from build123d import *

# Parameters (mm, degrees)
F1_DEPTH = 41.275
F2_W     = 82.55
F2_H     = 5.08
F3_DEPTH = 5.08
F4_W     = 92.71
F4_H     = 8.89
F5_DEPTH = 5.08
F6_W     = 5.0743944012
F6_H     = 7.62
F7_DEPTH = 6.35
F8_SIZE  = 1.27
F9_SIZE  = 3.048


with BuildPart() as f1:
    # F0 (on Front) → F1 (new body, symmetric)
    with BuildSketch(Plane.XZ):
        Polygon((-41.275, -3.81), (-41.275, 0), (-41.275, 5.08), (-46.355, 5.08), (-46.355, -3.81), align=None)
        Polygon((41.275, 0), (0, 0), (-41.275, 0), (-41.275, -3.81), (41.275, -3.81), align=None)
        Polygon((41.275, 5.08), (41.275, 0), (41.275, -3.81), (46.355, -3.81), (46.355, 5.08), align=None)
    extrude(amount=F1_DEPTH, both=True)

    # F2 (on face) → F3 (join)
    with BuildSketch(Plane.XZ.offset(41.275)):
        Polygon((-46.355, 5.08), (-46.355, -3.81), (46.355, -3.81), (46.355, 5.08), (41.275, 5.08), (41.275, 0), (-41.275, 0), (-41.275, 5.08), align=None)
        with Locations((0, 2.54)):
            Rectangle(F2_W, F2_H)
    extrude(amount=F3_DEPTH)

    # F4 (on face) → F5 (join)
    with BuildSketch(Plane(origin=(0, 41.275, 0), x_dir=(-1, 0, 0), z_dir=(0, 1, 0))):
        with Locations((0, 0.635)):
            Rectangle(F4_W, F4_H)
    extrude(amount=F5_DEPTH)

    # F6 (on face) → F7 (join)
    with BuildSketch(Plane.XZ.offset(46.355)):
        Rectangle(F6_W, F6_H)
    extrude(amount=F7_DEPTH)

    # F8
    f8_edges = [f1.edges().sort_by_distance(p)[0] for p in [
        (-2.537197, -49.53, 3.81),
        (2.537197, -49.53, 3.81),
        (0, -52.705, 3.81),
        (2.537197, -52.705, 0),
        (-2.537197, -52.705, 0),
    ]]
    chamfer(f8_edges, length=F8_SIZE)

    # F9
    f9_edges = [f1.edges().sort_by_distance(p)[0] for p in [
        (-41.275, 0, 5.08),
        (0, 41.275, 5.08),
        (0, -41.275, 5.08),
        (41.275, 0, 5.08),
    ]]
    chamfer(f9_edges, length=F9_SIZE)


solid = f1.part
Work out the finished part from the listing and answer in its coordinate system (mm). A direction names the side the tool comes from. Coordinates: 2 decimals unless noted, no trailing zeros. Write each loop counter-clockwise with the first axis right and the second up, starting at its lowest first coordinate (ties: lowest second). Pieces come first, ordered by that corner, then holes. Notation, with made-up numbers: M -5.75,9 L 26.25,9 A28 ccw 26.25,40 Z; hole C 18,58.25 d1. An arc over 180 degrees is marked long. Use one line per item in the form item = value. Start each with the question number.
1. Straight lines are drawn through the part: probe 1 along X at (y, z) = (15.5, 2) (3 decimals); probe 2 along Z at (x, y) = (-38, -16.5). For each, find the intervals that lie inside material, in ascending order. Write a range as from..to.
2. A tool of negligible diameter and unlimited length cuts with its end or side. For faces 1 (the face through (1, -1, 0)), 2 (the face through (-46.355, -1, 1)), 3 (the face through (2.537, -49, -1)), from which of +Z, -Z, +X, -X, +Y, -Y can it reach the whole face along a straight path? Write none if from no direction.
3. Each of these flat-tipped pins is pushed along its axis until it touches: P1, Ø2.5, axis at y = -49.5, z = -1.5, coming from the -X side; P2, Ø1.3, axis at x = 0.5, y = -50, coming from the +Z side; P3, Ø4, axis at y = -48.5, z = -1, coming from the +X side. Where does it stop, or does it pass through?
4. The part is cut by section A-A (y = -4). Give the vertices of the cut face in (x, z) (3 decimals), plus the area to 3 significant figures.
5. The mould has two halves that part along X. Classify faces 4 (the face through (0, -49, 3.81)), 5 (the face through (-2.537, -49, -1)), 6 (the face through (0.621, 42.778, 3.535)), 7 (the face through (-42.778, 0.621, 3.535)): released by +X, released by -X, zero draft, split by the parting line, or undercut.
Evaluation:
q1.probe_1 = -46.355..-41.275, 41.275..46.355
q1.probe_2 = -3.81..0
q2.face_1 = +Z
q2.face_2 = +Z, -Z, -X, +Y, -Y
q2.face_3 = +Z, -Z, +X, -Y
q3.P1 = -2.54
q3.P2 = 3.81
q3.P3 = 2.54
q4.outline = M -46.355,-3.81 L 46.355,-3.81 L 46.355,5.08 L 44.323,5.08 L 41.275,2.032 L 41.275,0 L -41.275,0 L -41.275,2.032 L -44.323,5.08 L -46.355,5.08 Z
q4.area = 396 mm^2
q5.face_4 = zero draft
q5.face_5 = released by -X
q5.face_6 = undercut
q5.face_7 = undercut
